Drawing for the job (mm, zero at the part's lowest x, y, z). Give positions to 0.01 mm unless a question says otherwise; leave off trailing zeros. Order: outer loops, then holes, each group sorted by start corner. A loop starts at its lowest first (then second) coordinate and runs counter-clockwise, first axis right, second up. Notation, with made-up numbers: (53, 33.5) - (111, 33.5) arc R32 ccw to (111, 60.5) - close; hole circle Ø9 at (37, -11.5). An arc over 180 degrees is marked (long way). One line per item, written item: value.
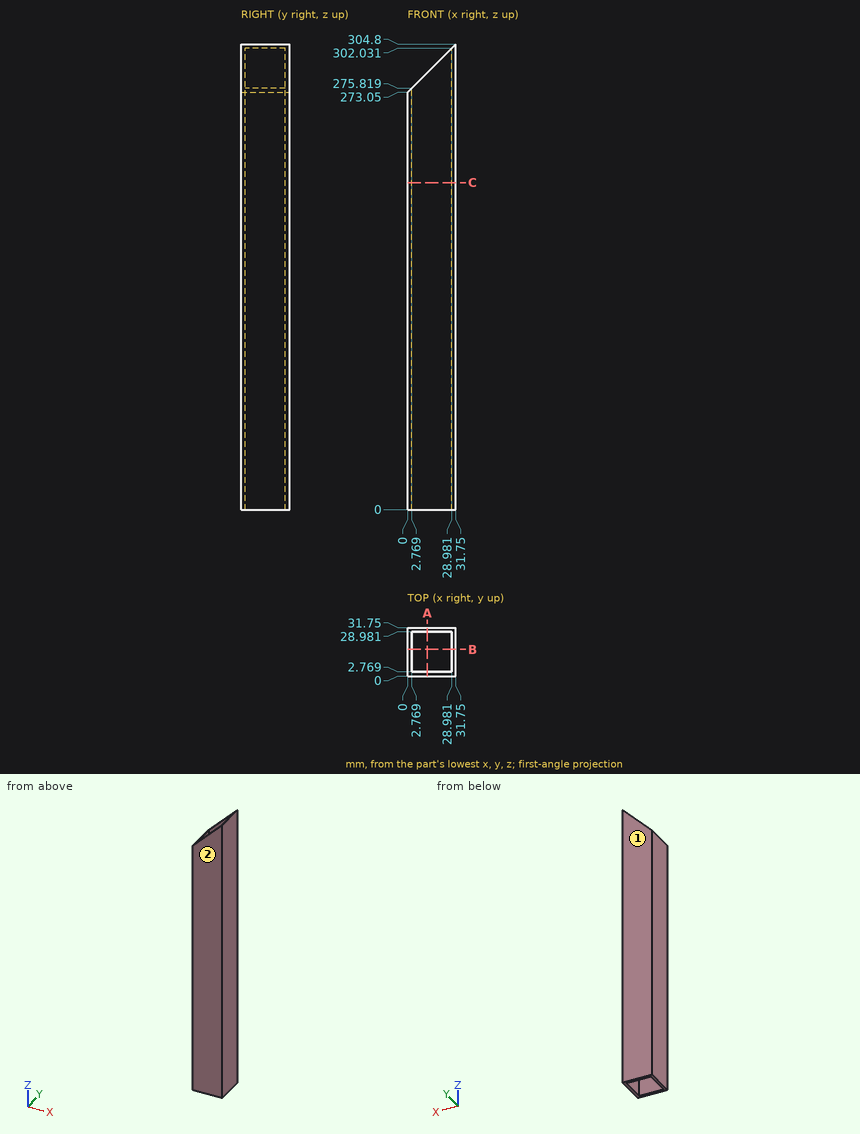
1) Drill centre lines: line 1 along Y through (x, z) = (19.5, 113.5); line 2 along X through (y, z) = (18, 285.5). Where is each one in solid material? Low to high. Write a range as from..to.
Outcome:
line 1: y = 0..2.77, 28.98..31.75
line 2: x = 28.98..31.75
2) Cut at B-B, the plane y = 17.5. Give the cut face in (x, z), then the cut area to 3 significant figures.
Outcome:
outline: (0, 0) - (2.77, 0) - (2.77, 275.82) - (0, 273.05) - close; (28.98, 0) - (31.75, 0) - (31.75, 304.8) - (28.98, 302.03) - close
area: 1,600 mm^2
3) Cut at C-C, the plane z = 214. Give the cut face in (x, y).
Outcome:
outline: (0, 0) - (31.75, 0) - (31.75, 31.75) - (0, 31.75) - close; hole (2.77, 2.77) - (28.98, 2.77) - (28.98, 28.98) - (2.77, 28.98) - close
4) Mould opens along Y. For the marked faces 1 and 2 say: released by +Y, released by -Y, zero draft, split by the parting line, or undercut.
Outcome:
face 1: released by +Y
face 2: released by -Y
5) Cut at A-A, the plane x = 13. Give the cut face in (y, z).
Outcome:
outline: (0, 0) - (2.77, 0) - (2.77, 286.05) - (0, 286.05) - close; (28.98, 0) - (31.75, 0) - (31.75, 286.05) - (28.98, 286.05) - close
